from build123d import *

# Parameters (mm, degrees)
SKETCH1_W           = 35
SKETCH1_H           = 35
BOSS_EXTRUDE1_DEPTH = 14
CUT_EXTRUDE1_DEPTH  = 57.868268832
SKETCH3_W           = 22
SKETCH3_H           = 31
CUT_EXTRUDE2_DEPTH  = 31
CUT_EXTRUDE3_DEPTH  = 57.868268832
FILLET1_R           = 2
CUT_EXTRUDE4_DEPTH  = 49.805737368
CUT_EXTRUDE5_DEPTH  = 49.805737368
SKETCH7_W           = 5.8
SKETCH7_H           = 2.6
BOSS_EXTRUDE2_DEPTH = 2.1
SKETCH8_W           = 5.8
SKETCH8_H           = 2.6
BOSS_EXTRUDE3_DEPTH = 2.1


with BuildPart() as part:
    # Sketch1 → Boss-Extrude1 (new, symmetric)
    with BuildSketch(Plane(origin=(0, 0, 0), x_dir=(0, 0, -1), z_dir=(1, 0, 0))):
        with Locations((-17.5, 17.5)):
            Rectangle(SKETCH1_W, SKETCH1_H)
    extrude(amount=BOSS_EXTRUDE1_DEPTH, both=True)

    # Sketch2 → Cut-Extrude1 (cut, through all)
    with BuildSketch(Plane.ZY.offset(14)):
        Polygon((35, 35), (6.4, 35), (35, 6.4), align=None)
    extrude(amount=-CUT_EXTRUDE1_DEPTH, mode=Mode.SUBTRACT)

    # Sketch3 → Cut-Extrude2 (cut)
    with BuildSketch(Plane(origin=(0, 35, 0), x_dir=(1, 0, 0), z_dir=(0, 1, 0))):
        with Locations((0, -19.5)):
            Rectangle(SKETCH3_W, SKETCH3_H)
    extrude(amount=-CUT_EXTRUDE2_DEPTH, mode=Mode.SUBTRACT)

    # Sketch4 → Cut-Extrude3 (cut, through all)
    with BuildSketch(Plane.ZY.offset(14)):
        Polygon((6.4, 35), (6.4, 28.6), (28.6, 6.4), (35, 6.4), align=None)
    extrude(amount=-CUT_EXTRUDE3_DEPTH, mode=Mode.SUBTRACT)

    # Fillet1
    fillet1_edges = [part.edges().sort_by_distance(p)[0] for p in [
        (12.5, 6.4, 35),
        (12.5, 35, 6.4),
        (-12.5, 6.4, 35),
        (-12.5, 35, 6.4),
    ]]
    fillet(fillet1_edges, radius=FILLET1_R)

    # Sketch5 → Cut-Extrude4 (cut, through all)
    with BuildSketch(Plane.XY.offset(4)):
        with BuildLine():
            Line((-3.3, 12.4), (-3.3, 22.7))
            ThreePointArc((-3.3, 22.7), (0, 26), (3.3, 22.7))
            Line((3.3, 22.7), (3.3, 12.4))
            ThreePointArc((3.3, 12.4), (0, 9.1), (-3.3, 12.4))
        make_face()
    extrude(amount=-CUT_EXTRUDE4_DEPTH, mode=Mode.SUBTRACT)

    # Sketch6 → Cut-Extrude5 (cut, through all)
    with BuildSketch(Plane(origin=(0, 4, 0), x_dir=(1, 0, 0), z_dir=(0, 1, 0))):
        with BuildLine():
            Line((3.3, -12.4), (3.3, -22.7))
            ThreePointArc((3.3, -22.7), (0, -26), (-3.3, -22.7))
            Line((-3.3, -22.7), (-3.3, -12.4))
            ThreePointArc((-3.3, -12.4), (0, -9.1), (3.3, -12.4))
        make_face()
    extrude(amount=-CUT_EXTRUDE5_DEPTH, mode=Mode.SUBTRACT)

    # Sketch7 → Boss-Extrude2 (add)
    with BuildSketch(Plane(origin=(0, 0, 0), x_dir=(-1, 0, 0), z_dir=(0, 0, -1))):
        with Locations((0, 31)):
            Rectangle(SKETCH7_W, SKETCH7_H)
        with Locations((0, 4)):
            Rectangle(SKETCH7_W, SKETCH7_H)
    extrude(amount=BOSS_EXTRUDE2_DEPTH)

    # Sketch8 → Boss-Extrude3 (add)
    with BuildSketch(Plane.XZ):
        with Locations((0, 31)):
            Rectangle(SKETCH8_W, SKETCH8_H)
        with Locations((0, 4)):
            Rectangle(SKETCH8_W, SKETCH8_H)
    extrude(amount=BOSS_EXTRUDE3_DEPTH)


solid = part.part
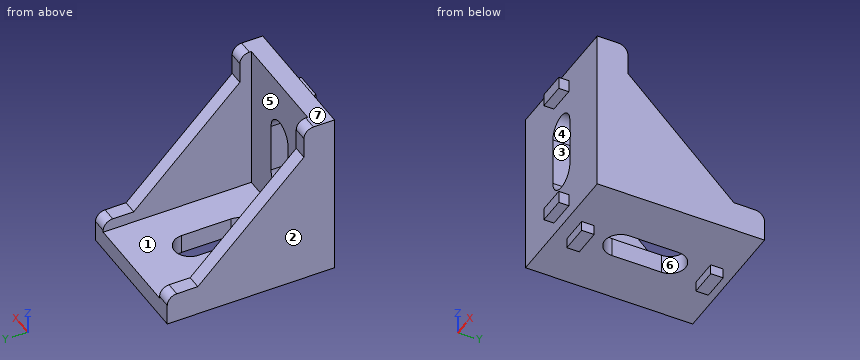
Could you check a few things on this model? Use its own coordinates, in mm. Face numbers are marked on the shaded views. A direction names the side the tool comes from. Give positions to 0.01 mm unless a question says otherwise; leave off trailing zeros. Order: outer loops, then holes, each group sorted by start corner. A loop starts at its lowest first (then second) coordinate and runs counter-clockwise, first axis right, second up.
Item 1: If we section it at C-C, the plane z = 10: Write out the boundary of the cut face in (x, y).
Item 2: If we section it at B-B, the plane x = 0: Count the separate pieces of the cut face and the enclosed holes in it, plus the area to 3 significant figures.
Item 3: If we mould it in two halves opening along Z, with no side actions, what happens to the marked faces 1, 2 and 3? For each: pulls with the +Z half, pulls with the -Z half, needs draft (parallel to the pull), parting line crosses it, or undercut.
Item 4: I'm going to push flat-ended pins straight in: pin 1 (1.7 mm diameter, centred on x = 0, y = -1.5, fed in from -Z); pin 2 (6 mm diameter, centred on x = -11, y = 24, fed in from -Z); pin 3 (3 mm diameter, centred on x = 3.5, z = 15, fed in from -Y); pin 4 (10 mm diameter, centred on x = 6.5, y = 8, fed in from +Z). Where does each tip first touch, or does it pass through?
Item 5: I need wall thicknesses on line 1 (X direction, y = 9.5, z = 16.5); line 2 (X direction, y = 3, z = 17); line 3 (Y direction, x = -10.25, z = 12). Which ranges of each line are inside material? Lowest first, please.
Item 6: For the marked faces 4, 5, 6 and 7, which set-ups out of +Z, -Z, +X, -X, +Y, -Y let a thin tool reach every point of the face, with its end or its side?
Item 7: If we section it at A-A, the plane y = 17.5: Write out the boundary of the cut face in (x, z), plus the area to 3 significant figures.
Item 8: If we section it at D-D, the plane y = 27.5: Write out the boundary of the cut face in (x, z), plus the area to 3 significant figures.
Values:
1. outline: (-14, 0) - (-2.26, 0) - (-2.26, 4) - (-11, 4) - (-11, 25) - (-14, 25) - close; (2.26, 0) - (14, 0) - (14, 25) - (11, 25) - (11, 4) - (2.26, 4) - close
2. separate pieces: 3
2. enclosed holes: 0
2. area: 151 mm2
3. face 1: pulls with the +Z half
3. face 2: needs draft
3. face 3: undercut
4. pin 1: stops at z = 2.7
4. pin 2: stops at z = 0
4. pin 3: stops at y = 0
4. pin 4: stops at z = 35
5. line 1: x = -14 to -11, 11 to 14
5. line 2: x = -14 to -3.3, 3.3 to 14
5. line 3: y = 0 to 4
6. face 4: +Y, -Y
6. face 5: +Z, +Y
6. face 6: +Z, -Z
6. face 7: +Z, +X, -X, +Y, -Y
7. outline: (-14, 0) - (-3.3, 0) - (-3.3, 4) - (-11, 4) - (-11, 17.5) - (-14, 17.5) - close; (3.3, 0) - (14, 0) - (14, 17.5) - (11, 17.5) - (11, 4) - (3.3, 4) - close
7. area: 167 mm2
8. outline: (-14, 0) - (14, 0) - (14, 7.5) - (11, 7.5) - (11, 4) - (-11, 4) - (-11, 7.5) - (-14, 7.5) - close
8. area: 133 mm2
